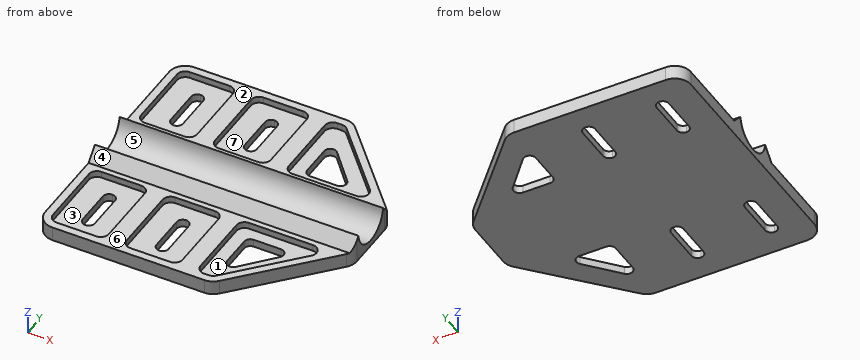
from build123d import *

# Parameters (mm, degrees)
F0_W         = 27.686
F0_H         = 19.685
F1_DEPTH     = 4.445
F4_DEPTH     = 82.55
F5_T4_DEPTH  = 82.55
F5_T9_DEPTH  = 82.55
F3_R         = 6.985
F6_DEPTH     = 101.6
F7_W         = 17.526
F7_H         = 25.4
F8_DEPTH     = 2.032
F9_R         = 2.54
F10_W        = 3.81
F10_H        = 15.24
F11_DEPTH    = 25.4
F12_R        = 1.90499
F13_T1_DEPTH = 29.845
F13_T3_DEPTH = 15.6401229428
F13_T5_DEPTH = 15.0634324568


# Not quite as in the source:
# - a fillet or chamfer that OpenCascade refuses, or shapes differently, is made with other operations: its cross-section is extruded or revolved along the edge and cut away or added
# - a fillet or chamfer is up to 0.001 mm smaller than in the source, because OpenCascade refuses the exact size


with BuildPart() as f1:
    # F0 (on Top) → F1 (new body)
    with BuildSketch(Plane.XY):
        Polygon((4.2753211141, 33.3069552488), (-50.5886788859, 33.3069552488), (-50.5886788859, -46.9570447512), (4.2753211141, -46.9570447512), (4.2753211141, -16.6675447512), (4.2753211141, 3.0174552488), align=None)
        Polygon((31.9613211141, 3.0174552488), (4.2753211141, 33.3069552488), (4.2753211141, 3.0174552488), align=None)
        with Locations((18.1183211141, -6.8250447512)):
            Rectangle(F0_W, F0_H)
        Polygon((4.2753211141, -16.6675447512), (4.2753211141, -46.9570447512), (31.9613211141, -16.6675447512), align=None)
    extrude(amount=F1_DEPTH)

    # F3 (on face) → F4 (join)
    with BuildSketch(Plane.YZ.offset(31.9613211141)):
        with BuildLine():
            Line((-1.4368910785, 4.445), (-12.2131984238, 4.445))
            ThreePointArc((-12.2131984238, 4.445), (-6.8250447512, 1.905), (-1.4368910785, 4.445))
        make_face()
        with BuildLine():
            ThreePointArc((-1.4368910785, 4.445), (-0.2513669981, 6.5284357306), (0.1599552488, 8.89))
            ThreePointArc((0.1599552488, 8.89), (-9.1866090205, 15.4636777531), (-12.2131984238, 4.445))
            Line((-12.2131984238, 4.445), (-1.4368910785, 4.445))
        make_face()
    extrude(amount=-F4_DEPTH)

    # F5: chamfer of 7.62 on 2 edges, made by hand


with BuildPart() as f5_tool2:
    # F5_s3 → F5_t4 (new body)
    with BuildSketch(Plane.YZ.offset(31.9613211141)):
        with BuildLine():
            Line((3.9242683255, 4.2209526948), (-0.0694446449, 8.550803314))
            Line((-0.0694446449, 8.550803314), (-0.2213483693, 8.5630922738))
            ThreePointArc((-0.2213483693, 8.5630922738), (-0.4679887951, 6.3855514916), (-1.554450795, 4.5419818182))
            Line((-1.554450795, 4.5419818182), (-1.4368910785, 4.2926))
            ThreePointArc((-1.4368910785, 4.2926), (1.2436886235, 4.2926), (3.9242683255, 4.0685526948))
            Line((3.9242683255, 4.0685526948), (3.9242683255, 4.2209526948))
        make_face()
    extrude(amount=-F5_T4_DEPTH)

    split(bisect_by=Plane(origin=(18.9157105891, 17.2898319012, 0), x_dir=(0, 0, 1), z_dir=(-0.7381168756, -0.6746728674, 0)), keep=Keep.TOP)


with BuildPart() as f1_1:
    add(f1.part)

    # F5_t1: union F5_tool2
    add(f5_tool2.part)


with BuildPart() as f5_tool7:
    # F5_s8 → F5_t9 (new body)
    with BuildSketch(Plane.YZ.offset(-50.5886788859)):
        with BuildLine():
            Line((-17.5743578278, 4.2209526948), (-13.5806448574, 8.550803314))
            Line((-13.5806448574, 8.550803314), (-13.4287411331, 8.5630922738))
            ThreePointArc((-13.4287411331, 8.5630922738), (-13.1821007073, 6.3855514916), (-12.0956387073, 4.5419818182))
            Line((-12.0956387073, 4.5419818182), (-12.2131984238, 4.2926))
            ThreePointArc((-12.2131984238, 4.2926), (-14.8937781258, 4.2926), (-17.5743578278, 4.0685526948))
            Line((-17.5743578278, 4.0685526948), (-17.5743578278, 4.2209526948))
        make_face()
    extrude(amount=F5_T9_DEPTH)

    split(bisect_by=Plane(origin=(25.7132835648, -23.5031271159, 0), x_dir=(0, 0, 1), z_dir=(-0.7381168756, 0.6746728674, 0)), keep=Keep.TOP)


with BuildPart() as f1_2:
    add(f1_1.part)

    # F5_t6: union F5_tool7
    add(f5_tool7.part)

    # F3 (on face) → F6 (cut)
    with BuildSketch(Plane.YZ.offset(31.9613211141)):
        with Locations((-6.8250447512, 8.89)):
            Circle(F3_R)
    extrude(amount=-F6_DEPTH, mode=Mode.SUBTRACT)

    # F7 (on face) → F8 (cut)
    with BuildSketch(Plane.XY.offset(4.445)):
        with Locations((-39.3872788859, -31.8059447512)):
            Rectangle(F7_W, F7_H)
        with Locations((-16.2732788859, -31.8186447512)):
            Rectangle(F7_W, F7_H)
        Polygon((26.4173608001, -19.1186447512), (-1.9222788859, -19.1186447512), (-1.9222788859, -44.5186447512), (3.2005893116, -44.5186447512), align=None)
        Polygon((3.2005893116, 30.8685552488), (-1.9222788859, 30.8685552488), (-1.9222788859, 5.4685552488), (26.4173608001, 5.4685552488), align=None)
        with Locations((-39.3872788859, 18.1558552488)):
            Rectangle(F7_W, F7_H)
        with Locations((-16.2732788859, 18.1685552488)):
            Rectangle(F7_W, F7_H)
    extrude(amount=-F8_DEPTH, mode=Mode.SUBTRACT)

    # F9
    f9_edges = [f1_2.edges().sort_by_distance(p)[0] for p in [
        (-48.150279, -19.105945, 3.429),
        (-48.150279, 30.855855, 3.429),
        (-25.036279, 30.868555, 3.429),
        (-1.922279, 30.868555, 3.429),
        (3.200589, 30.868555, 3.429),
        (-1.922279, -19.118645, 3.429),
        (-25.036279, -19.118645, 3.429),
        (-30.624279, 30.855855, 3.429),
        (-7.510279, 30.868555, 3.429),
        (26.417361, -19.118645, 3.429),
        (-7.510279, -19.118645, 3.429),
        (-30.624279, -19.105945, 3.429),
        (3.200589, -44.518645, 3.429),
        (-7.510279, -44.518645, 3.429),
        (-30.624279, -44.505945, 3.429),
        (-7.510279, 5.468555, 3.429),
        (-30.624279, 5.455855, 3.429),
        (-48.150279, 5.455855, 3.429),
        (-48.150279, -44.505945, 3.429),
        (-25.036279, -44.518645, 3.429),
        (-1.922279, -44.518645, 3.429),
        (-1.922279, 5.468555, 3.429),
        (-25.036279, 5.468555, 3.429),
        (26.417361, 5.468555, 3.429),
    ]]
    fillet(f9_edges, radius=F9_R)

    # F10 (on face) → F11 (cut)
    with BuildSketch(Plane.XY.offset(4.445)):
        with Locations((-39.3872788859, -31.8059447512)):
            Rectangle(F10_W, F10_H)
        with Locations((-16.2732788859, -31.8186447512)):
            Rectangle(F10_W, F10_H)
        Polygon((16.8492179688, -22.7416258461), (2.1748828364, -22.7416258461), (2.1748828364, -39.307281707), align=None)
        Polygon((16.8492179688, 9.0915363437), (2.1748828364, 25.6571922047), (2.1748828364, 9.0915363437), align=None)
        with Locations((-16.2732788859, 18.1685552488)):
            Rectangle(F10_W, F10_H)
        with Locations((-39.3872788859, 18.1558552488)):
            Rectangle(F10_W, F10_H)
    extrude(amount=-F11_DEPTH, mode=Mode.SUBTRACT)

    # F12 (radius 1.905 in the source; OpenCascade refuses exactly that, so slightly less here)
    f12_edges = [f1_2.edges().sort_by_distance(p)[0] for p in [
        (-41.292279, -24.185945, 1.2065),
        (-37.482279, -24.185945, 1.2065),
        (-14.368279, -24.198645, 1.2065),
        (16.849218, -22.741626, 1.2065),
        (-14.368279, 25.788555, 1.2065),
        (-37.482279, 25.775855, 1.2065),
        (-18.178279, -24.198645, 1.2065),
        (2.174883, -22.741626, 1.2065),
        (-18.178279, 25.788555, 1.2065),
        (-41.292279, 25.775855, 1.2065),
        (2.174883, 25.657192, 1.2065),
        (-41.292279, -39.425945, 1.2065),
        (-18.178279, -39.438645, 1.2065),
        (-41.292279, 10.535855, 1.2065),
        (-18.178279, 10.548555, 1.2065),
        (2.174883, 9.091536, 1.2065),
        (-14.368279, -39.438645, 1.2065),
        (-37.482279, -39.425945, 1.2065),
        (-14.368279, 10.548555, 1.2065),
        (-37.482279, 10.535855, 1.2065),
        (16.849218, 9.091536, 1.2065),
        (2.174883, -39.307282, 1.2065),
    ]]
    fillet(f12_edges, radius=F12_R)

    # F13: fillet of radius 5.08 on 6 edges, made by hand

    # F13_s2 → F13_t1 (cut)
    with BuildSketch(Plane.XY.offset(-12.7)):
        with BuildLine():
            ThreePointArc((-50.5886788859, -41.8770447512), (-49.1007813343, -45.4691471996), (-45.5086788859, -46.9570447512))
            Line((-45.5086788859, -46.9570447512), (-50.5886788859, -46.9570447512))
            Line((-50.5886788859, -46.9570447512), (-50.5886788859, -41.8770447512))
        make_face()
        with BuildLine():
            ThreePointArc((-45.5086788859, 33.3069552488), (-49.1007813343, 31.8190576973), (-50.5886788859, 28.2269552488))
            Line((-50.5886788859, 28.2269552488), (-50.5886788859, 33.3069552488))
            Line((-50.5886788859, 33.3069552488), (-45.5086788859, 33.3069552488))
        make_face()
    extrude(amount=F13_T1_DEPTH, mode=Mode.SUBTRACT)

    # F13_s4 → F13_t3 (cut)
    with BuildSketch(Plane.XY.offset(-5.5975614714)):
        with BuildLine():
            ThreePointArc((2.0362965256, -46.9570447512), (4.0851403599, -46.5255540759), (5.7859302534, -45.3043829175))
            Line((5.7859302534, -45.3043829175), (4.2753211141, -46.9570447512))
            Line((4.2753211141, -46.9570447512), (2.0362965256, -46.9570447512))
        make_face()
        with BuildLine():
            ThreePointArc((2.0362965256, 33.3069552488), (4.0851403599, 32.8754645736), (5.7859302534, 31.6542934152))
            Line((5.7859302534, 31.6542934152), (4.2753211141, 33.3069552488))
            Line((4.2753211141, 33.3069552488), (2.0362965256, 33.3069552488))
        make_face()
    extrude(amount=F13_T3_DEPTH, mode=Mode.SUBTRACT)

    # F13_s6 → F13_t5 (cut)
    with BuildSketch(Plane.XY.offset(-4.9296716098)):
        with BuildLine():
            ThreePointArc((31.9613211141, -14.6956761073), (31.6170649489, -16.5339172044), (30.630954842, -18.1230142736))
            Line((30.630954842, -18.1230142736), (31.9613211141, -16.6675447512))
            Line((31.9613211141, -16.6675447512), (31.9613211141, -14.6956761073))
        make_face()
        with BuildLine():
            ThreePointArc((30.630954842, 4.4729247713), (31.6170649489, 2.8838277021), (31.9613211141, 1.0455866049))
            Line((31.9613211141, 1.0455866049), (31.9613211141, 3.0174552488))
            Line((31.9613211141, 3.0174552488), (30.630954842, 4.4729247713))
        make_face()
    extrude(amount=F13_T5_DEPTH, mode=Mode.SUBTRACT)


solid = f1_2.part
Here's how the part is built. I have some questions about the finished solid (model axes, mm). Face numbers are marked on the shaded views. A direction names the side the tool comes from. Coordinates: 2 decimals unless noted, no trailing zeros. Write each loop counter-clockwise with the first axis right and the second up, starting at its lowest first coordinate (ties: lowest second). Pieces come first, ordered by that corner, then holes.
Item 1: Will these pins go through, and if not, where does the flat tip stop? pin 1 (12.5 mm diameter, centred on x = 7.5, y = 19.5, fed in from +Z) (3 decimals); pin 2 (1.6 mm diameter, centred on y = 14.5, z = 3.5, fed in from +X); pin 3 (1.6 mm diameter, centred on y = 18.5, z = 3, fed in from +X).
Item 2: On a 3-axis mill with a long thin cutter (end or side, diameter ignored), from which of +Z, -Z, +X, -X, +Y, -Y can I reach the whole of each face in a straight line? I mean the marked faces 5, 6 and 7. Say none if no direction works.
Item 3: I want a section at B-B on x = -5. Write out the boundary of the cut face in (y, z) (3 decimals).
Item 4: If we mould it in two halves opening along Y, with no side actions, what happens to the marked faces 1, 2, 3 and 4? For each: +Y half, -Y half, draft (parallel to the pull), parting line (faces both ways), or undercut.
Item 5: If I drill on line 1 (Y direction, x = -16.5, z = 1.75); line 2 (X direction, y = -21, z = 3.5); line 3 (Z direction, x = -12, y = -43), over which ranges is the centre line in solid material (lowest first)?
Item 6: I want a section at D-D on y = -6. Write out the boundary of the cut face in (x, z).
Item 7: I want a section at C-C on x = 9.5. Write out the boundary of the cut face in (y, z) (3 decimals).
Item 8: I want a section at A-A on y = 17. Write out the boundary of the cut face in (x, z) (3 decimals).
Findings below:
1. pin 1: stops at z = 4.445
1. pin 2: stops at x = 22.2
1. pin 3: stops at x = 18.54
2. face 5: +Z, +X, -X
2. face 6: +Z, +X, -X, -Y
2. face 7: +Z
3. outline: (-46.957, 0) - (33.307, 0) - (33.307, 4.445) - (3.718, 4.445) - (0.137, 8.327) arc R6.985 cw to (-13.787, 8.327) - (-17.368, 4.445) - (-46.957, 4.445) - close
4. face 1: undercut
4. face 2: draft
4. face 3: undercut
4. face 4: -Y half
5. line 1: y = -46.96 to -39.43, -24.21 to 10.56, 25.78 to 33.31
5. line 2: x = -50.59 to -48.07, -30.71 to -24.95, -7.6 to -1.84, 23.11 to 28
5. line 3: z = 0 to 2.41
6. outline: (-50.59, 0) - (31.96, 0) - (31.96, 1.95) - (-50.59, 1.95) - close
7. outline: (-41.241, 0) - (-31.038, 0) - (-31.038, 2.413) - (-37.627, 2.413) - (-37.627, 4.445) - (-41.241, 4.445) - close; (-22.742, 0) - (9.092, 0) - (9.092, 2.413) - (5.469, 2.413) - (5.469, 4.445) - (3.718, 4.445) - (0.137, 8.327) arc R6.985 cw to (-13.787, 8.327) - (-17.368, 4.445) - (-19.119, 4.445) - (-19.119, 2.413) - (-22.742, 2.413) - close; (17.388, 0) - (27.591, 0) - (27.591, 4.445) - (23.977, 4.445) - (23.977, 2.413) - (17.388, 2.413) - close
8. outline: (-50.589, 0) - (-41.292, 0) - (-41.292, 2.413) - (-48.15, 2.413) - (-48.15, 4.445) - (-50.589, 4.445) - close; (-37.482, 0) - (-18.178, 0) - (-18.178, 2.413) - (-25.036, 2.413) - (-25.036, 4.445) - (-30.624, 4.445) - (-30.624, 2.413) - (-37.482, 2.413) - close; (-14.368, 0) - (2.175, 0) - (2.175, 2.413) - (-1.922, 2.413) - (-1.922, 4.445) - (-7.51, 4.445) - (-7.51, 2.413) - (-14.368, 2.413) - close; (9.844, 0) - (19.181, 0) - (19.181, 4.445) - (15.877, 4.445) - (15.877, 2.413) - (9.844, 2.413) - close
